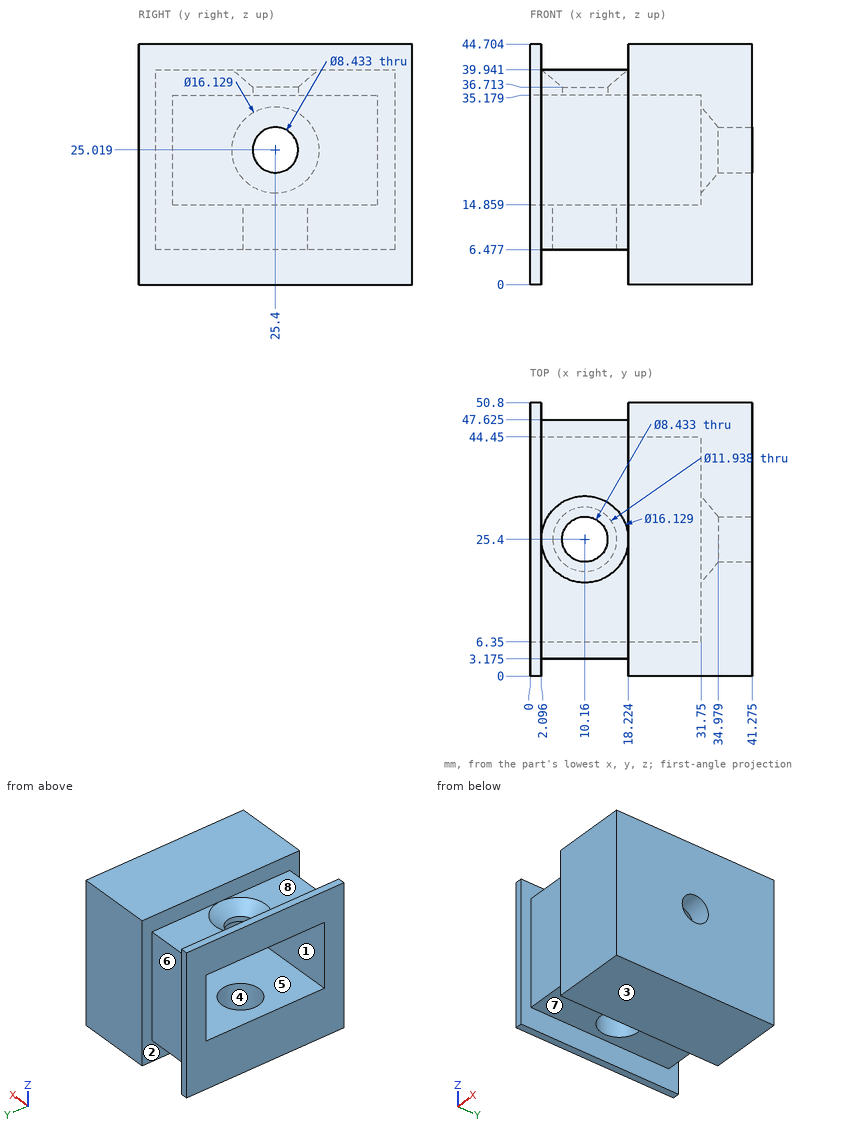
Verification items for this drawing (mm, ordinates from the low corner). A direction names the side the tool comes from. Give positions to 0.01 mm unless a question says otherwise; leave off trailing zeros. Return JSON: item names as keys, results as strings. Group by question number.
1. Go/stop test with flat-tipped pins: pin 1 (5 mm diameter, centred on x = 11.5, z = 36.5, fed in from -Y) (1 decimal); pin 2 (5 mm diameter, centred on y = 12, z = 27, fed in from -X); pin 3 (9.5 mm diameter, centred on y = 25.4, z = 25.019, fed in from -X). Record where each tip stops, or that it passes through.
2. Tool access check on the marked faces 4, 5, 6, 7 and 8. Record the directions out of +Z, -Z, +X, -X, +Y, -Y that give a thin tool (end or side, any length) a straight path to the whole face; none if there is none.
3. Thickness scan on L1, parallel to X at y = 25, z = 8 (1 decimal); L2, parallel to Y at x = 10.16, z = 12.75 (1 decimal); L3, parallel to Y at x = 18.5, z = 20.5. Record the ranges inside material, lowest first.
4. Mould release check, pull along Z, two halves, no side actions. Record for the marked faces 1, 2 and 3: released by +Z, released by -Z, zero draft, split by the parting line, or undercut.
Return value:
{
 "1": {"pin 1": "y = 3.2", "pin 2": "x = 31.75", "pin 3": "x = 34.53"},
 "2": {"face 4": "-Z", "face 5": "-X", "face 6": "+Z, -Z, +Y", "face 7": "-Z, +Y, -Y", "face 8": "+Z, +Y, -Y"},
 "3": {"L1": "0 to 4.2, 16.1 to 41.3", "L2": "3.2 to 19.4, 31.4 to 47.6", "L3": "0 to 6.35, 44.45 to 50.8"},
 "4": {"face 1": "undercut", "face 2": "zero draft", "face 3": "released by -Z"}
}
